Answer from the drawing. Dimensions are ordinates in mm from the lowest x, y and z of the part. A direction names the side the tool comes from. Give positions to 0.01 mm unless a question says otherwise; leave off trailing zeros. Loops run counter-clockwise (first coordinate to the right, second up) from the corner with the lowest first, then second, coordinate; pieces in that order, holes last.
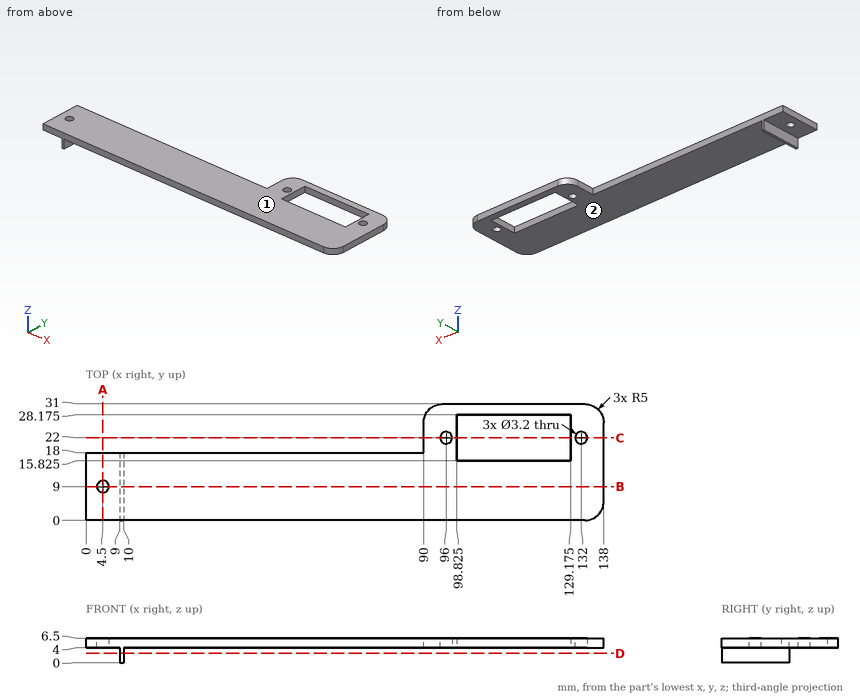
Item 1: Find section B-B, the plane y = 9. Write down the section's boundary in (x, z), plus the area to 3 significant figures.
Item 2: Consider line 1 (X direction, y = 20, z = 6.25) (3 decimals); line 2 (X direction, y = 3, z = 1.75); line 3 (Y direction, x = 116, z = 5.5) (3 decimals). Determine where each line is inside the solid, lowest interval first.
Item 3: Find section D-D, the plane z = 2.5. Write down the section's boundary in (x, y), plus the area to 3 significant figures.
Item 4: For the marked faces 1 and 2, determine the directions among +Z, -Z, +X, -X, +Y, -Y from which every point of the face is accessible in a straight line to the end or side of a thin tool.
Item 5: Flat-ended cylindrical pins translate along their axes: pin 1 Ø1.2 at (y, z) = (21, 6) entering from -X; pin 2 Ø4.5 at (x, y) = (6, 7) entering from -Z; pin 3 Ø1 at (y, z) = (15.5, 3) entering from -X; pin 4 Ø1.9 at (x, y) = (4.5, 9) entering from +Z. Find the tip coordinate at first contact, or state that the pin passes through.
Item 6: Find section C-C, the plane y = 22. Write down the section's boundary in (x, z) (3 decimals), plus the area to 3 significant figures.
Item 7: Find section A-A, the plane x = 4.5. Write down the section's boundary in (y, z), plus the area to 3 significant figures.
Ans:
1. outline: (0, 4) - (2.9, 4) - (2.9, 6.5) - (0, 6.5) - close; (6.1, 4) - (9, 4) - (9, 0) - (10, 0) - (10, 4) - (138, 4) - (138, 6.5) - (6.1, 6.5) - close
1. area: 341 mm2
2. line 1: x = 90 to 98.825, 129.175 to 138
2. line 2: x = 9 to 10
2. line 3: y = 0 to 15.825, 28.175 to 31
3. outline: (9, 0) - (10, 0) - (10, 18) - (9, 18) - close
3. area: 18.0 mm2
4. face 1: +Z, +X, -X, +Y, -Y
4. face 2: -Z, +X, +Y, -Y
5. pin 1: stops at x = 90
5. pin 2: stops at z = 4
5. pin 3: stops at x = 9
5. pin 4: passes through
6. outline: (90, 4) - (94.4, 4) - (94.4, 6.5) - (90, 6.5) - close; (97.6, 4) - (98.825, 4) - (98.825, 6.5) - (97.6, 6.5) - close; (129.175, 4) - (130.4, 4) - (130.4, 6.5) - (129.175, 6.5) - close; (133.6, 4) - (138, 4) - (138, 6.5) - (133.6, 6.5) - close
6. area: 28.1 mm2
7. outline: (0, 4) - (7.4, 4) - (7.4, 6.5) - (0, 6.5) - close; (10.6, 4) - (18, 4) - (18, 6.5) - (10.6, 6.5) - close
7. area: 37.0 mm2
